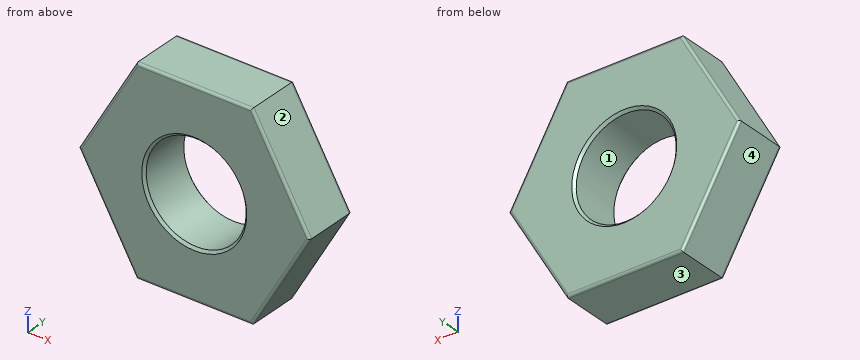
```python
from build123d import *

# Parameters (mm, degrees)
SKETCH1_R           = 2
BOSS_EXTRUDE1_DEPTH = 2.15
FILLET1_R           = 0.1
CHAMFER1_SIZE       = 0.1


with BuildPart() as part:
    # Sketch1 → Boss-Extrude1 (new body)
    with BuildSketch(Plane(origin=(0, 0, 0), x_dir=(1, 0, 0), z_dir=(0, 1, 0))):
        Polygon((-2.309401077, 4), (2.309401077, 4), (4.618802154, 0), (2.309401077, -4), (-2.309401077, -4), (-4.618802154, 0), align=None)
        with Locations(Location((0, 0, 0), (0, 0, 90))):
            Circle(SKETCH1_R, mode=Mode.SUBTRACT)
    extrude(amount=BOSS_EXTRUDE1_DEPTH)

    # Fillet1
    fillet1_edges = [part.edges().sort_by_distance(p)[0] for p in [
        (3.464101615, 2.15, -2),
        (3.464101615, 2.15, 2),
        (0, 2.15, 4),
        (-3.464101615, 2.15, 2),
        (-3.464101615, 2.15, -2),
        (-3.464101615, 0, 2),
        (0, 0, 4),
        (3.464101615, 0, 2),
        (3.464101615, 0, -2),
        (0, 0, -4),
        (-3.464101615, 0, -2),
        (0, 2.15, -4),
    ]]
    fillet(fillet1_edges, radius=FILLET1_R)

    # Chamfer1
    chamfer1_edges = [part.edges().sort_by_distance(p)[0] for p in [
        (0, 0, 2),
        (0, 2.15, 2),
    ]]
    chamfer(chamfer1_edges, length=CHAMFER1_SIZE)


solid = part.part
```
Build history of the part. All positions in model axes, mm. Face numbers are marked on the shaded views. Round coordinates to 2 decimals unless told otherwise and drop trailing zeros. Loops run counter-clockwise (first coordinate to the right, second up) from the corner with the lowest first, then second, coordinate; pieces in that order, holes last.
Item 1: Saw through at B-B (y = 0.9). List the corners of the cut face in (x, z).
Item 2: Pin check, flat tip, straight feed: P1, Ø1, axis at y = 2, z = -2.5, coming from the +X side. Stop position of the tip, or through.
Item 3: Saw through at A-A (x = 0). List the corners of the cut face in (y, z).
Item 4: Drill centre lines: line 1 along X through (y, z) = (0.75, 1.25); line 2 along Z through (x, y) = (0.25, 1.2); line 3 along X through (y, z) = (2, 3). Where is each one in solid material? Low to high.
Item 5: Two-plate mould, pull along X, no slides. Class the marked faces 1, 2, 3 and 4: released by +X, released by -X, zero draft, split by the parting line, or undercut.
Worked answers:
1. outline: (-4.62, 0) - (-2.31, -4) - (2.31, -4) - (4.62, 0) - (2.31, 4) - (-2.31, 4) - close; hole circle Ø4 at (0, 0)
2. P1: stops at x = 3.46
3. outline: (0, -3.9) arc R0.1 ccw to (0.1, -4) - (2.05, -4) arc R0.1 ccw to (2.15, -3.9) - (2.15, -2.1) - (2.05, -2) - (0.1, -2) - (0, -2.1) - close; (0, 2.1) - (0.1, 2) - (2.05, 2) - (2.15, 2.1) - (2.15, 3.9) arc R0.1 ccw to (2.05, 4) - (0.1, 4) arc R0.1 ccw to (0, 3.9) - close
4. line 1: x = -3.9 to -1.56, 1.56 to 3.9
4. line 2: z = -4 to -1.98, 1.98 to 4
4. line 3: x = -2.89 to 2.89
5. face 1: undercut
5. face 2: released by +X
5. face 3: zero draft
5. face 4: released by -X
